from build123d import *

# Parameters (mm, degrees)
F1_R     = 6
F2_DEPTH = 40
F0_R     = 10
F3_DEPTH = 5
F4_SIZE  = 0.5
F5_SIZE  = 1.5


# Not quite as in the source:
# - the program builds the solid bodies; features that only make, move or delete a surface that nothing else refers to are left out


with BuildPart() as f2:
    # F1 (on face) → F2 (new body)
    with BuildSketch(Plane.XY):
        Circle(F1_R)
    extrude(amount=F2_DEPTH)

    # F0 (on Top) → F3 (join)
    with BuildSketch(Plane.XY):
        Circle(F0_R)
    extrude(amount=-F3_DEPTH)

    # F4
    f4_edges = [f2.edges().sort_by_distance(p)[0] for p in [
        (-10, 0, 0),
        (-10, 0, -5),
    ]]
    chamfer(f4_edges, length=F4_SIZE)

    # F5
    f5_edges = [f2.edges().sort_by_distance(p)[0] for p in [
        (-6, 0, 40),
    ]]
    chamfer(f5_edges, length=F5_SIZE)


solid = f2.part
Build history of the part. All positions in model axes, mm. A direction names the side the tool comes from. Round coordinates to 2 decimals unless told otherwise and drop trailing zeros. Write each loop counter-clockwise with the first axis right and the second up, starting at its lowest first coordinate (ties: lowest second). Pieces come first, ordered by that corner, then holes. Notation, with made-up numbers: M 11.25,29 L 70.25,29 A7 cw 70.25,40 Z; hole C 40.25,-29 d8. An arc over 180 degrees is marked long. Answer as a JSON object with one key per item and string values. Group by question number.
(1) Drill centre lines: L1, parallel to Z at x = 2.75, y = -7; L2, parallel to Y at x = 2.5, z = 33; L3, parallel to X at y = 5, z = 13.5. Where is each one in solid material? Low to high.
(2) Cut at C-C (z = 3). Give the cut face in (x, y), and give its area (3 significant figures).
(3) Which spindle directions (+Z, -Z, +X, -X, +Y, -Y) get a long thin tool onto all of the face, cutting with end or side? Do faces 1 (the flat face through (-0.1, -6.2, 0)), 2 (the flat face through (0, 0, -5)). Say none if no direction does.
(4) Cut at A-A (y = 0). Give the cut face in (x, z).
(5) Cut at D-D (z = -2). Give the cut face in (x, y).
(6) Flat gauge pins, fed straight in: pin 1 (6 mm diameter, centred on y = -2.5, z = 0.5, fed in from -X); pin 2 (1 mm diameter, centred on y = -5.5, z = 4, fed in from -X); pin 3 (5 mm diameter, centred on x = 6.5, z = 12.5, fed in from -Y); pin 4 (1.5 mm diameter, centred on x = 4, z = 28.5, fed in from +Y). Where does each tip first touch, or does it go through?
Responses:
{
 "1": {"L1": "z = -5 to 0", "L2": "y = -5.45 to 5.45", "L3": "x = -3.32 to 3.32"},
 "2": {"outline": "C 0,0 d12", "area": "113 mm2"},
 "3": {"face 1": "+Z", "face 2": "-Z, +X, -X, +Y, -Y"},
 "4": {"outline": "M -10,-4.5 L -9.5,-5 L 9.5,-5 L 10,-4.5 L 10,-0.5 L 9.5,0 L 6,0 L 6,38.5 L 4.5,40 L -4.5,40 L -6,38.5 L -6,0 L -9.5,0 L -10,-0.5 Z"},
 "5": {"outline": "C 0,0 d20"},
 "6": {"pin 1": "stops at x = -10", "pin 2": "stops at x = -3.32", "pin 3": "stops at y = -4.47", "pin 4": "stops at y = 5.04"}
}
